from build123d import *

# Parameters (mm, degrees)
SKETCH1_R                                            = 10
BOSS_EXTRUDE1_DEPTH                                  = 10
SKETCH1_3_R                                          = 10
BOSS_EXTRUDE2_DEPTH                                  = 20
SKETCH1_4_W                                          = 15
SKETCH1_4_H                                          = 22
BOSS_EXTRUDE3_DEPTH                                  = 50
CSK_FOR_M8_HEX_SOCKET_COUNTERSUNK_CAP_SC_D           = 9
CSK_FOR_M8_HEX_SOCKET_COUNTERSUNK_CAP_SC_CSINK_D     = 17.92
CSK_FOR_M8_HEX_SOCKET_COUNTERSUNK_CAP_SC_CSINK_ANGLE = 90
TAP_DRILL_FOR_M8_TAP1_D                              = 12
TAP_DRILL_FOR_M8_TAP1_DEPTH                          = 10
TAP_DRILL_FOR_M8_TAP1_TIP                            = 3.464101615


with BuildPart() as part:
    # Sketch1 → Boss-Extrude1 (new body)
    with BuildSketch(Plane(origin=(0, 0, 0), x_dir=(1, 0, 0), z_dir=(0, 1, 0))):
        Polygon((0, 5), (0, 0), (70, 0), (70, 35), (35, 35), (35, 13), (35, 5), align=None)
        with Locations(Location((55, 20, 0), (0, 0, 270))):
            Circle(SKETCH1_R, mode=Mode.SUBTRACT)
    extrude(amount=BOSS_EXTRUDE1_DEPTH)

    # Sketch1_3 → Boss-Extrude2 (add)
    with BuildSketch(Plane(origin=(0, 0, 0), x_dir=(1, 0, 0), z_dir=(0, 1, 0))):
        Polygon((0, 35), (0, 5), (35, 5), (35, 13), (20, 13), (20, 35), align=None)
        with Locations(Location((55, 20, 0), (0, 0, 270))):
            Circle(SKETCH1_3_R)
    extrude(amount=BOSS_EXTRUDE2_DEPTH)

    # Sketch1_4 → Boss-Extrude3 (add)
    with BuildSketch(Plane(origin=(0, 0, 0), x_dir=(1, 0, 0), z_dir=(0, 1, 0))):
        with Locations((27.5, 24)):
            Rectangle(SKETCH1_4_W, SKETCH1_4_H)
    extrude(amount=BOSS_EXTRUDE3_DEPTH)

    # CSK for M8 Hex Socket Countersunk Cap Sc (through all)
    with Locations(Plane(origin=(55, 20, -20), x_dir=(0, 0, 1), z_dir=(0, 1, 0))):
        with Locations((0, 0)):
            CounterSinkHole(CSK_FOR_M8_HEX_SOCKET_COUNTERSUNK_CAP_SC_D / 2, CSK_FOR_M8_HEX_SOCKET_COUNTERSUNK_CAP_SC_CSINK_D / 2, counter_sink_angle=CSK_FOR_M8_HEX_SOCKET_COUNTERSUNK_CAP_SC_CSINK_ANGLE)

    # Sketch5 → CBORE for M6 Hex Socket Head Cap Screw1 (revolve, cut)
    with BuildSketch(Plane(origin=(10, 20, -25), x_dir=(0, 0, 1), z_dir=(1, 0, 0))):
        Polygon((0, 0), (0, 11.922753981), (3.2, 10), (3.2, 6.4), (5.5, 6.4), (5.5, 2), (7.5, 0), align=None)
    revolve(axis=Axis((10, 26.35, -25), (0, -1, 0)), mode=Mode.SUBTRACT)

    # Tap Drill for M8 Tap1
    with Locations(Plane(origin=(35, 40, -25), x_dir=(0, 0, 1), z_dir=(1, 0, 0))):
        with Locations((0, 0)):
            Hole(TAP_DRILL_FOR_M8_TAP1_D / 2, depth=TAP_DRILL_FOR_M8_TAP1_DEPTH)
            with Locations((0, 0, -(TAP_DRILL_FOR_M8_TAP1_DEPTH + TAP_DRILL_FOR_M8_TAP1_TIP / 2))):  # 120° drill point
                Cone(0, TAP_DRILL_FOR_M8_TAP1_D / 2, TAP_DRILL_FOR_M8_TAP1_TIP, mode=Mode.SUBTRACT)


solid = part.part
Work out the finished part from the listing and answer in its coordinate system (mm). A direction names the side the tool comes from. Coordinates: 2 decimals unless noted, no trailing zeros. Loops run counter-clockwise (first coordinate to the right, second up) from the corner with the lowest first, then second, coordinate; pieces in that order, holes last. Notation, with made-up numbers: M 68,70 L 123,70 A20 ccw 123,80 Z; hole C 30,15 d1. An arc over 180 degrees is marked long. Answer in a Markdown table with one row per item. Add a question column.
1. The mould has two halves that part along X. Classify faces 1 (the flat face through (0, 10, -18)), 2 (the flat face through (61, 20, -27)), 3 (the conical face through (58.98, 15.76, -22.54)): pulls with the +X half, pulls with the -X half, needs draft (parallel to the pull), parting line crosses it, or undercut.
2. Consider L1, parallel to X at y = 11, z = -20; L2, parallel to X at y = 11.45, z = -25; L3, parallel to Z at x = 10, y = 15.85. Determine where each line is inside the solid, lowest interval first.
3. Find section C-C, the plane x = 30. Write down the section's boundary in (y, z), then the cut area to 3 significant figures.
4. Find section A-A, the plane y = 12. Write down the section's boundary in (x, z).
5. Flat-ended cylindrical pins translate along their axes: P1, Ø5, axis at x = 10, z = -25, coming from the +Y side; P2, Ø1.5, axis at x = 47.5, z = -26, coming from the +Y side; P3, Ø2, axis at x = 8.5, z = -30.5, coming from the +Y side. Find the tip coordinate at first contact, or state that the pin passes through.
6. A tool of negligible diameter and unlimited length cuts with its end or side. For faces 4 (the flat face through (35, 25, -23)), 5 (the cylindrical face through (29.93, 43.65, -20.24)), 6 (the cylindrical face through (46.128, 14.93, -15.386)), 7 (the flat face through (13, 20, -17)), 8 (the flat face through (27, 35, -13)), from which of +Z, -Z, +X, -X, +Y, -Y can it reach the whole face along a straight path? Write none if from no direction.
7. Find section B-B, the plane x = 55. Write down the section's boundary in (y, z).
8. Find section D-D, the plane z = -4. Write down the section's boundary in (x, y), then the cut area to 3 significant figures.
Reported:
| question | item | result |
|---|---|---|
| 1 | face 1 | pulls with the -X half |
| 1 | face 2 | needs draft |
| 1 | face 3 | undercut |
| 2 | L1 | x = 0 to 35, 45 to 50.5, 59.5 to 65 |
| 2 | L2 | x = 0 to 6.8, 13.2 to 35, 46.34 to 63.66 |
| 2 | L3 | z = -35 to -30.5, -19.5 to -5 |
| 3 | outline | M 0,-35 L 50,-35 L 50,-13 L 20,-13 L 20,-5 L 10,-5 L 10,0 L 0,0 Z; hole C 40,-25 d12 |
| 3 | area | 1,200 mm^2 |
| 4 | outline | M 0,-35 L 35,-35 L 35,-5 L 0,-5 Z; C 55,-20 d20; hole C 10,-25 d6.4; hole C 55,-20 d9 |
| 5 | P1 | stops at y = 9.58 |
| 5 | P2 | stops at y = 20 |
| 5 | P3 | stops at y = 19.2 |
| 6 | face 4 | +Z, -Z, +Y |
| 6 | face 5 | +X |
| 6 | face 6 | +Y |
| 6 | face 7 | +Z, -X, +Y |
| 6 | face 8 | +Z, +X, -X, +Y |
| 7 | outline | M 0,-35 L 10,-35 L 10,-30 L 20,-30 L 20,-28.96 L 15.54,-24.5 L 0,-24.5 Z; M 0,-15.5 L 15.54,-15.5 L 20,-11.04 L 20,-10 L 10,-10 L 10,0 L 0,0 Z |
| 8 | outline | M 0,0 L 70,0 L 70,10 L 0,10 Z |
| 8 | area | 700 mm^2 |
